The model under review builds one solid part; all positions refer to its coordinate system, in mm. A direction names the side the tool comes from. Round coordinates to 2 decimals unless told otherwise and drop trailing zeros. Order: outer loops, then holes, each group sorted by start corner. A loop starts at its lowest first (then second) coordinate and runs counter-clockwise, first axis right, second up. Notation, with made-up numbers: (5, -15.75) -> (31, -15.75) arc R27 cw to (31, 4.25) -> close; hole circle Ø9 at (63, 23). An arc over 180 degrees is marked (long way). Use a Markdown table: item, result. Add a question column.
```python
from build123d import *

# Parameters (mm, degrees)
SKETCH1_W           = 39
SKETCH1_H           = 45
BOSS_EXTRUDE1_DEPTH = 12.5
SKETCH2_R           = 4.05
CUT_EXTRUDE1_DEPTH  = 61.846117378
SKETCH3_W           = 50
SKETCH3_H           = 50
BOSS_EXTRUDE2_DEPTH = 5.5
BOSS_EXTRUDE3_START = -10
BOSS_EXTRUDE3_DEPTH = 5
LPATTERN1_COUNT     = 2
LPATTERN1_PITCH     = 14
FILLET1_R           = 5
SKETCH5_R           = 1.6
CUT_EXTRUDE2_DEPTH  = 76.175212005
FILLET2_R           = 20
CUT_EXTRUDE3_DEPTH  = 70.381643826
CUT_EXTRUDE4_START  = -1
SKETCH7_W           = 39
SKETCH7_H           = 50.063664736
SKETCH7_R           = 11
SKETCH7_W_2         = 11
SKETCH7_H_2         = 11
CUT_EXTRUDE4_DEPTH  = 1
SKETCH8_W           = 25
SKETCH8_H           = 5
SKETCH8_W_2         = 5
SKETCH8_H_2         = 25
BOSS_EXTRUDE4_DEPTH = 0.5
SKETCH9_W           = 34.8
SKETCH9_H           = 11.25
CUT_EXTRUDE5_DEPTH  = 0.2


with BuildPart() as part:
    # Sketch1 → Boss-Extrude1 (new body)
    with BuildSketch(Plane(origin=(0, 0, 0), x_dir=(1, 0, 0), z_dir=(0, 1, 0))):
        with Locations((19.5, 22.5)):
            Rectangle(SKETCH1_W, SKETCH1_H)
    extrude(amount=BOSS_EXTRUDE1_DEPTH)

    # Sketch2 → Cut-Extrude1 (cut, through all)
    with BuildSketch(Plane(origin=(0, 12.5, 0), x_dir=(1, 0, 0), z_dir=(0, 1, 0))):
        with Locations(Location((19.5, 15, 0), (0, 0, 270))):
            Circle(SKETCH2_R)
    extrude(amount=-CUT_EXTRUDE1_DEPTH, mode=Mode.SUBTRACT)

    # Sketch3 → Boss-Extrude2 (add)
    with BuildSketch(Plane(origin=(0, 0, -45), x_dir=(-1, 0, 0), z_dir=(0, 0, -1))):
        with Locations((-4, 14.75)):
            Rectangle(SKETCH3_W, SKETCH3_H)
    extrude(amount=BOSS_EXTRUDE2_DEPTH)

    # Sketch4 → Boss-Extrude3 (add)
    with BuildSketch(Plane(origin=(39, 0, 0), x_dir=(0, 0, -1), z_dir=(1, 0, 0)).offset(BOSS_EXTRUDE3_START)):
        Polygon((33, 12.5), (45, 24.5), (45, 12.5), align=None)
    boss_extrude3 = extrude(amount=-BOSS_EXTRUDE3_DEPTH)

    # LPattern1: Boss-Extrude3 ×2
    with Locations(*[(-i * LPATTERN1_PITCH, 0, 0) for i in range(1, LPATTERN1_COUNT)]):
        add(boss_extrude3)

    # Fillet1
    fillet1_edges = [part.edges().sort_by_distance(p)[0] for p in [
        (26.5, 12.5, -33),
        (26.5, 24.5, -45),
        (12.5, 12.5, -33),
        (12.5, 24.5, -45),
    ]]
    fillet(fillet1_edges, radius=FILLET1_R)

    # Sketch5 → Cut-Extrude2 (cut, through all)
    with BuildSketch(Plane(origin=(0, 0, -50.5), x_dir=(-1, 0, 0), z_dir=(0, 0, -1))):
        with Locations((-22, 32.75)):
            Circle(SKETCH5_R)
        with Locations((14, 32.75)):
            Circle(SKETCH5_R)
        with Locations((14, -3.25)):
            Circle(SKETCH5_R)
        with Locations((-22, -3.25)):
            Circle(SKETCH5_R)
    extrude(amount=-CUT_EXTRUDE2_DEPTH, mode=Mode.SUBTRACT)

    # Fillet2
    # the kernel refuses this fillet: 20 mm, written as the material it takes off along each edge
    with BuildSketch(Plane(origin=(0, -50, 0), x_dir=(0, 0, -1), z_dir=(0, 1, 0)), Plane(origin=(39, -50, 0), x_dir=(-1, 0, 0), z_dir=(0, 1, 0))) as fillet2_piece_1:
        with BuildLine():
            CenterArc((FILLET2_R, -FILLET2_R), FILLET2_R, 90, 90)
            Line((0, -FILLET2_R), (0, 0))
            Line((0, 0), (FILLET2_R, 0))
        make_face()
    extrude(amount=112.5, mode=Mode.SUBTRACT)

    # Sketch6 → Cut-Extrude3 (cut, through all)
    with BuildSketch(Plane(origin=(0, 12.5, 0), x_dir=(1, 0, 0), z_dir=(0, 1, 0))):
        with BuildLine():
            Line((7, 20), (7, 28.347560338))
            Line((7, 28.347560338), (15.5, 28.347560338))
            Line((15.5, 28.347560338), (15.5, 25.246950766))
            ThreePointArc((15.5, 25.246950766), (10.417048938, 21.204836823), (8.5, 15))
            ThreePointArc((8.5, 15), (7.383077909, 17.389923373), (7, 20))
        make_face()
        with BuildLine():
            Line((23.5, 25.246950766), (23.5, 28.347560338))
            Line((23.5, 28.347560338), (32, 28.347560338))
            Line((32, 28.347560338), (32, 20))
            ThreePointArc((32, 20), (31.605614865, 17.768951725), (30.47026085, 15.808317311))
            ThreePointArc((30.47026085, 15.808317311), (28.348679441, 21.534590434), (23.5, 25.246950766))
        make_face()
    extrude(amount=-CUT_EXTRUDE3_DEPTH, mode=Mode.SUBTRACT)

    # Sketch7 → Cut-Extrude4 (cut)
    with BuildSketch(Plane.XZ.offset(CUT_EXTRUDE4_START)):
        with Locations((19.5, -19.968167632)):
            Rectangle(SKETCH7_W, SKETCH7_H)
        with Locations(Location((19.5, -15, 0), (0, 0, 180))):
            Circle(SKETCH7_R, mode=Mode.SUBTRACT)
        with Locations((10, -37.501795484)):
            Rectangle(SKETCH7_W_2, SKETCH7_H_2, mode=Mode.SUBTRACT)
        with Locations((29, -37.501795484)):
            Rectangle(SKETCH7_W_2, SKETCH7_H_2, mode=Mode.SUBTRACT)
    extrude(amount=CUT_EXTRUDE4_DEPTH, mode=Mode.SUBTRACT)

    # Sketch8 → Boss-Extrude4 (add)
    with BuildSketch(Plane(origin=(0, 0, -50.5), x_dir=(-1, 0, 0), z_dir=(0, 0, -1))):
        with Locations((-4, 32.75)):
            Rectangle(SKETCH8_W, SKETCH8_H)
        with Locations((14, 14.75)):
            Rectangle(SKETCH8_W_2, SKETCH8_H_2)
        with Locations((-4, -3.25)):
            Rectangle(SKETCH8_W, SKETCH8_H)
        with Locations((-22, 14.75)):
            Rectangle(SKETCH8_W_2, SKETCH8_H_2)
    extrude(amount=BOSS_EXTRUDE4_DEPTH)

    # Sketch9 → Cut-Extrude5 (cut)
    with BuildSketch(Plane.XY.offset(-45)):
        with Locations((11.6, -4.625)):
            Rectangle(SKETCH9_W, SKETCH9_H)
    extrude(amount=-CUT_EXTRUDE5_DEPTH, mode=Mode.SUBTRACT)


solid = part.part
```
Q1. Add section A-A (y = -3.25). Write out the cut boundary in (x, z), then the cut area to 3 significant figures.
Q2. Add section D-D (x = -14). Write out the cut boundary in (y, z), then the cut area to 3 significant figures.
Q3. Add section C-C (z = -24.5). Write out the cut boundary in (x, y).
Q4. Machinability: for faces 4 (the flat face through (32, 7, -24)), 5 (the flat face through (10, 0, -38)), 6 (the flat face through (19, 12.5, -23)), which of the approach directions +Z, -Z, +X, -X, +Y, -Y give a long, thin tool a straight path to every point of the face, cutting with its end or side? Answer none if there is none.
Q5. Wall thickness on line 1 (Y direction, x = -14, z = -48.85); line 2 (X direction, y = -3, z = -49); line 3 (X direction, y = 11.5, z = -44.5): over which ranges is each line inside the solid? List them lowest first. Write a range as [from, to].
Q6. Insertion check: pin 1 (1 mm diameter, centred on y = 7, z = -7, fed in from -X); pin 2 (8 mm diameter, centred on x = 6, z = -8, fed in from +Y); pin 3 (12 mm diameter, centred on x = 31, y = 19, fed in from -Z); pin 4 (1 mm diameter, centred on y = -1, z = -39.5, fed in from +X). Each pin has a flat end and moves straight along its axis. Give the tip position at first contact, or say it passes through.
Q7. Mouldability with a two-part tool opening along Z and no side actions: class faces 1 (the flat face through (4, 33, -51)), 2 (the cylindrical face through (21.26, 31.33, -47.79)), 3 (the cylindrical face through (31.616, 6.83, -17.799)) as pulls with the +Z half, pulls with the -Z half, needs draft (parallel to the pull), parting line crosses it, or undercut.
Q8. Add section B-B (y = 9). Write out the cut boundary in (x, z).
Report:
| question | item | result |
|---|---|---|
| 1 | outline | (-21, -50.5) -> (-15.6, -50.5) -> (-15.6, -45) -> (-21, -45) -> close; (-12.4, -50.5) -> (-8.5, -50.5) -> (-8.5, -51) -> (16.5, -51) -> (16.5, -50.5) -> (20.4, -50.5) -> (20.4, -45.2) -> (-5.8, -45.2) -> (-5.8, -45) -> (-12.4, -45) -> close; (23.6, -50.5) -> (29, -50.5) -> (29, -45.2) -> (23.6, -45.2) -> close |
| 1 | area | 246 mm² |
| 2 | outline | (-10.25, -50.5) -> (-4.85, -50.5) -> (-4.85, -45) -> (-10.25, -45) -> close; (-1.65, -50.5) -> (2.25, -50.5) -> (2.25, -51) -> (27.25, -51) -> (27.25, -50.5) -> (31.15, -50.5) -> (31.15, -45) -> (-1.65, -45) -> close; (34.35, -50.5) -> (39.75, -50.5) -> (39.75, -45) -> (34.35, -45) -> close |
| 2 | area | 252 mm² |
| 3 | outline | (0, 1) -> (7, 1) -> (7, 12.5) -> (0, 12.5) -> close; (13.95, 0) -> (25.05, 0) -> (25.05, 12.5) -> (13.95, 12.5) -> close; (32, 1) -> (39, 1) -> (39, 12.5) -> (32, 12.5) -> close |
| 4 | face 4 | +Y, -Y |
| 4 | face 5 | +Z, +X, -X, -Y |
| 4 | face 6 | +Z, +Y |
| 5 | line 1 | y = [-10.25, -4.85], [-1.65, 31.15], [34.35, 39.75] |
| 5 | line 2 | x = [-21, -15.58], [-12.42, 20.42], [23.58, 29] |
| 5 | line 3 | x = [0, 39] |
| 6 | pin 1 | stops at x = 4.39 |
| 6 | pin 2 | stops at y = 12.5 |
| 6 | pin 3 | stops at z = -50.5 |
| 6 | pin 4 | passes through |
| 7 | face 1 | pulls with the -Z half |
| 7 | face 2 | needs draft |
| 7 | face 3 | undercut |
| 8 | outline | (-21, -50.5) -> (-16.5, -50.5) -> (-16.5, -51) -> (-11.5, -51) -> (-11.5, -50.5) -> (19.5, -50.5) -> (19.5, -51) -> (24.5, -51) -> (24.5, -50.5) -> (29, -50.5) -> (29, -45) -> (39, -45) -> (39, -20) arc R20 ccw to (19.5, -0.01) arc R20 ccw to (0, -20) -> (0, -45) -> (-21, -45) -> close; hole (7, -28.35) -> (15.5, -28.35) -> (15.5, -25.25) arc R11 cw to (8.5, -15) arc R9.08 ccw to (7, -20) -> close; hole circle Ø8.1 at (19.5, -15); hole (23.5, -28.35) -> (32, -28.35) -> (32, -20) arc R6.51 ccw to (30.47, -15.81) arc R11 cw to (23.5, -25.25) -> close |
